```python
from build123d import *

# Parameters (mm, degrees)
F0_W     = 80
F0_H     = 500
F1_DEPTH = 80
F2_R     = 20
F3_W     = 20.159984
F3_H     = 52.525729
F4_DEPTH = 35
F5_W     = 18.923229
F5_H     = 40.931299
F6_DEPTH = 35


with BuildPart() as f1:
    # F0 (on Top) → F1 (new body)
    with BuildSketch(Plane.XY):
        Rectangle(F0_W, F0_H)
    extrude(amount=F1_DEPTH)

    # F2
    f2_edges = [f1.edges().sort_by_distance(p)[0] for p in [
        (-40, 0, 0),
        (40, 0, 0),
        (40, 0, 80),
        (-40, 0, 80),
    ]]
    fillet(f2_edges, radius=F2_R)

    # F3 (on face) → F4 (join)
    with BuildSketch(Plane.XY.offset(80)):
        with Locations((0, 206.395387)):
            Rectangle(F3_W, F3_H)
    extrude(amount=F4_DEPTH)

    # F5 (on face) → F6 (join)
    with BuildSketch(Plane(origin=(0, 0, 0), x_dir=(1, 0, 0), z_dir=(0, 0, -1))):
        with Locations((9.461614, -220.531561)):
            Rectangle(F5_W, F5_H)
    extrude(amount=F6_DEPTH)


solid = f1.part
```
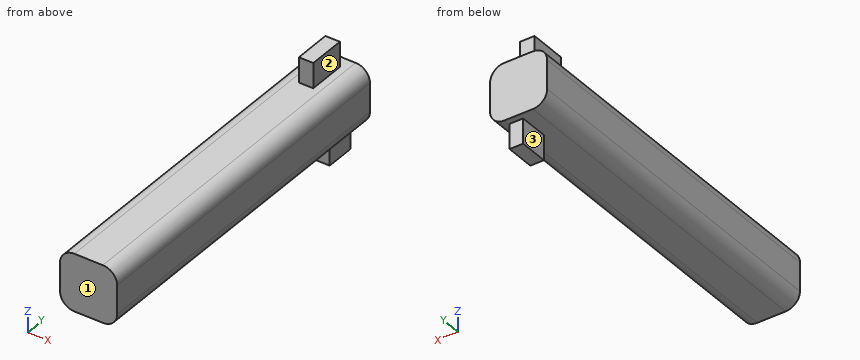
Model file for the job. Use its own axes, mm. Face numbers are marked on the shaded views. A direction names the side the tool comes from. Coordinates: 2 decimals unless noted, no trailing zeros. Write each loop counter-clockwise with the first axis right and the second up, starting at its lowest first coordinate (ties: lowest second). Pieces come first, ordered by that corner, then holes. Notation, with made-up numbers: (62.5, -26.5) - (76.5, -26.5) arc R15 cw to (76.5, 1.5) - close; hole circle Ø6 at (-9, 18.5). An arc over 180 degrees is marked (long way). Use a Markdown table: item, result. Add a question column.
Item 1: Drop flat-ended pins along their axis: pin 1 (4 mm diameter, centred on x = 28.5, y = 185, fed in from +Z); pin 2 (3 mm diameter, centred on x = 30, y = 128, fed in from +Z); pin 3 (12 mm diameter, centred on x = -7, y = 33.5, fed in from -Z). Give the stop position or say it passes through.
Item 2: 3-axis set-ups, long thin cutter, end or side, ignore diameter. For the marked faces 1, 2 and 3: which of +Z, -Z, +X, -X, +Y, -Y reach the whole face in a straight line?
Item 3: Band-saw the part on B-B, the plane z = 84.5. Write the cut outline in (x, y), and give its area (3 significant figures).
Item 4: Band-saw the part on C-C, the plane x = 27.5. Write the cut outline in (y, z), and give its area (3 significant figures).
Item 5: Drill centre lines: line 1 along X through (y, z) = (208, 105); line 2 along Z through (x, y) = (11.5, -75.5); line 3 along Y through (x, z) = (-10, 92). Where is each one in solid material? Low to high.
Item 6: Band-saw the part on A-A, the plane y = 123.5. Write the cut outline in (x, z), and give its area (3 significant figures).
A:
| question | item | result |
|---|---|---|
| 1 | pin 1 | stops at z = 78.91 |
| 1 | pin 2 | stops at z = 78.1 |
| 1 | pin 3 | stops at z = 0 |
| 2 | face 1 | +Z, -Z, +X, -X, -Y |
| 2 | face 2 | +Z, +X, +Y, -Y |
| 2 | face 3 | -Z, -X, +Y, -Y |
| 3 | outline | (-10.08, 180.13) - (10.08, 180.13) - (10.08, 232.66) - (-10.08, 232.66) - close |
| 3 | area | 1,060 mm² |
| 4 | outline | (-250, 1.46) - (250, 1.46) - (250, 78.54) - (-250, 78.54) - close |
| 4 | area | 38,500 mm² |
| 5 | line 1 | x = -10.08 to 10.08 |
| 5 | line 2 | z = 0 to 80 |
| 5 | line 3 | y = 180.13 to 232.66 |
| 6 | outline | (-40, 20) arc R20 ccw to (-20, 0) - (20, 0) arc R20 ccw to (40, 20) - (40, 60) arc R20 ccw to (20, 80) - (-20, 80) arc R20 ccw to (-40, 60) - close |
| 6 | area | 6,060 mm² |
